Here's how the part is built. I have some questions about the finished solid (model axes, mm). Coordinates: 2 decimals unless noted, no trailing zeros. Loops run counter-clockwise (first coordinate to the right, second up) from the corner with the lowest first, then second, coordinate; pieces in that order, holes last. Notation, with made-up numbers: (24.5, -4) - (53.5, -4) arc R26 cw to (53.5, 25) - close; hole circle Ø5 at (16.25, 67). An arc over 180 degrees is marked (long way). Use a Markdown table: item, result.
```python
from build123d import *

# Parameters (mm, degrees)
SKETCH1_R           = 2
BOSS_EXTRUDE3_DEPTH = 5
FILLET9_R           = 10
FILLET10_R          = 3
FILLET11_R          = 3
FILLET12_R          = 3
FILLET13_R          = 0.5


with BuildPart() as part:
    # Sketch1 → Boss-Extrude3 (new body)
    with BuildSketch(Plane(origin=(0, 0, 0), x_dir=(1, 0, 0), z_dir=(0, 1, 0))):
        with BuildLine():
            Line((-4.046119318, 54.590604732), (-4.046119318, -7.195574606))
            ThreePointArc((-4.046119318, -7.195574606), (-11.635335702, -12.035866866), (-15.176119318, -20.311583503))
            ThreePointArc((-15.176119318, -20.311583503), (-15.239015435, -21.109389908), (-15.26, -21.909396551))
            ThreePointArc((-15.26, -21.909396551), (-15.239086668, -22.708042569), (-15.17640413, -23.504499555))
            Line((-15.17640413, -23.504499555), (-16.906872391, -23.686379161))
            ThreePointArc((-16.906872391, -23.686379161), (-18.44583537, -24.118938522), (-19.753766933, -25.038084689))
            ThreePointArc((-19.753766933, -25.038084689), (-19.56295199, -26.067629867), (-19.318516287, -27.085777598))
            ThreePointArc((-19.318516287, -27.085777598), (-17.749810888, -27.393475541), (-16.167960532, -27.162685373))
            Line((-16.167960532, -27.162685373), (-14.513122101, -26.624995641))
            ThreePointArc((-14.513122101, -26.624995641), (-14.246436916, -27.378091201), (-13.940703236, -28.116197446))
            ThreePointArc((-13.940703236, -28.116197446), (-13.596759365, -28.837290674), (-13.215547785, -29.539395055))
            Line((-13.215547785, -29.539395055), (-14.722432114, -30.409395176))
            ThreePointArc((-14.722432114, -30.409395176), (-15.952407023, -31.430510437), (-16.773411552, -32.802175926))
            ThreePointArc((-16.773411552, -32.802175926), (-16.180339688, -33.665100824), (-15.542918581, -34.49580411))
            ThreePointArc((-15.542918581, -34.49580411), (-13.984682857, -34.138850219), (-12.633461458, -33.284616422))
            Line((-12.633461458, -33.284616422), (-11.340389428, -32.120328997))
            ThreePointArc((-11.340389428, -32.120328997), (-10.790448835, -32.699845394), (-10.210932372, -33.249785918))
            ThreePointArc((-10.210932372, -33.249785918), (-9.603428978, -33.768642793), (-8.969603297, -34.25499435))
            Line((-8.969603297, -34.25499435), (-9.99234972, -35.66268407))
            ThreePointArc((-9.99234972, -35.66268407), (-10.700662735, -37.095795135), (-10.892781095, -38.682806536))
            ThreePointArc((-10.892781095, -38.682806536), (-9.999999818, -39.229903609), (-9.079809202, -39.729526311))
            ThreePointArc((-9.079809202, -39.729526311), (-7.80147625, -38.769641154), (-6.914522249, -37.439668504))
            Line((-6.914522249, -37.439668504), (-6.20680051, -35.850099247))
            ThreePointArc((-6.20680051, -35.850099247), (-5.468694229, -36.155832838), (-4.715598637, -36.422517933))
            ThreePointArc((-4.715598637, -36.422517933), (-3.94957857, -36.649423393), (-3.172733001, -36.835927528))
            Line((-3.172733001, -36.835927528), (-3.534499379, -38.53790452))
            ThreePointArc((-3.534499379, -38.53790452), (-3.598676752, -40.135213481), (-3.128689936, -41.66316212))
            ThreePointArc((-3.128689936, -41.66316212), (-2.09056923, -41.799833318), (-1.046718412, -41.881986139))
            ThreePointArc((-1.046718412, -41.881986139), (-0.269323601, -40.48514257), (6.05e-07, -38.909395406))
            Line((6.05e-07, -38.909395406), (5.43e-07, -37.169395268))
            ThreePointArc((5.43e-07, -37.169395268), (0.798647238, -37.14848194), (1.595104896, -37.085799334))
            ThreePointArc((1.595104896, -37.085799334), (2.387189815, -36.981519365), (3.172731623, -36.835927821))
            Line((3.172731623, -36.835927821), (3.534497981, -38.537904817))
            ThreePointArc((3.534497981, -38.537904817), (4.1255531, -40.023222459), (5.176380106, -41.22791215))
            ThreePointArc((5.176380106, -41.22791215), (6.180339749, -40.930525784), (7.167359489, -40.581003755))
            ThreePointArc((7.167359489, -40.581003755), (7.309397542, -38.988728703), (6.914523355, -37.439668011))
            Line((6.914523355, -37.439668011), (6.206801502, -35.850098805))
            ThreePointArc((6.206801502, -35.850098805), (6.927895349, -35.506154662), (7.630000317, -35.124942746))
            ThreePointArc((7.630000317, -35.124942746), (8.311191417, -34.707508302), (8.969602158, -34.254995178))
            ThreePointArc((8.969602158, -34.254995178), (10.210932755, -33.249785573), (11.340390155, -32.12032819))
            ThreePointArc((11.340390155, -32.12032819), (11.859247485, -31.512824296), (12.345599442, -30.87899807))
            ThreePointArc((12.345599442, -30.87899807), (12.7981126, -30.220587353), (13.215547081, -29.539396275))
            ThreePointArc((13.215547081, -29.539396275), (13.940703446, -28.116196975), (14.513122436, -26.624994609))
            ThreePointArc((14.513122436, -26.624994609), (14.740028108, -25.8589739), (14.926532387, -25.08212767))
            ThreePointArc((14.926532387, -25.08212767), (13.533608818, -14.858931995), (5.953880682, -7.858811478))
            Line((5.953880682, -7.858811478), (5.953880682, 54.590604732))
            ThreePointArc((5.953880682, 54.590604732), (-0.92910996, 71.20761409), (-17.546119318, 78.090604732))
            Line((-17.546119318, 78.090604732), (-17.546119318, 68.090604732))
            ThreePointArc((-17.546119318, 68.090604732), (-8.000177772, 64.136546278), (-4.046119318, 54.590604732))
        make_face()
        with Locations((0, -21.909395268)):
            Circle(SKETCH1_R, mode=Mode.SUBTRACT)
        with Locations((-12.546119318, 72.402117863)):
            Circle(SKETCH1_R, mode=Mode.SUBTRACT)
    extrude(amount=BOSS_EXTRUDE3_DEPTH)

    # Fillet9
    fillet9_edges = [part.edges().sort_by_distance(p)[0] for p in [
        (5.953880682, 2.5, 7.858811478),
    ]]
    fillet(fillet9_edges, radius=FILLET9_R)

    # Fillet10
    fillet10_edges = [part.edges().sort_by_distance(p)[0] for p in [
        (-4.046119318, 2.5, 7.195574606),
    ]]
    fillet(fillet10_edges, radius=FILLET10_R)

    # Fillet11
    fillet11_edges = [part.edges().sort_by_distance(p)[0] for p in [
        (-17.546119318, 2.5, -78.090604732),
    ]]
    fillet(fillet11_edges, radius=FILLET11_R)

    # Fillet12
    fillet12_edges = [part.edges().sort_by_distance(p)[0] for p in [
        (-17.546119318, 2.5, -68.090604732),
    ]]
    fillet(fillet12_edges, radius=FILLET12_R)

    # Fillet13
    fillet13_edges = [part.edges().sort_by_distance(p)[0] for p in [
        (7.167359489, 2.5, 40.581003755),
        (5.176380106, 2.5, 41.22791215),
        (-1.046718412, 2.5, 41.881986139),
        (-3.128689936, 2.5, 41.66316212),
        (-9.079809202, 2.5, 39.729526311),
        (-10.892781095, 2.5, 38.682806536),
        (-15.542918581, 2.5, 34.49580411),
        (-16.773411552, 2.5, 32.802175926),
        (-19.318516287, 2.5, 27.085777598),
        (-19.753766933, 2.5, 25.038084689),
    ]]
    fillet(fillet13_edges, radius=FILLET13_R)


solid = part.part
```
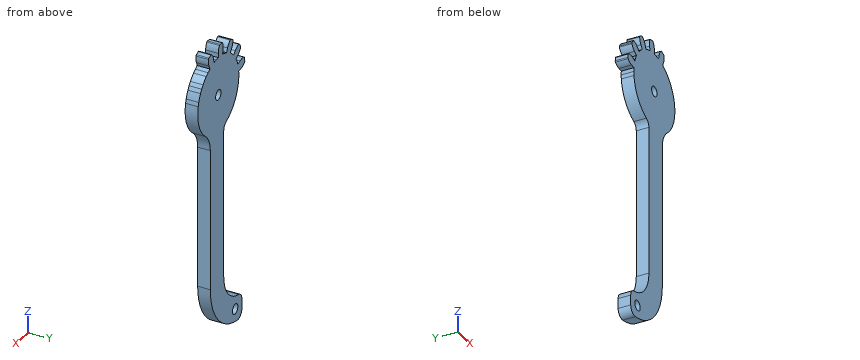
Q1. I want a section at B-B, the plane z = -42.5. Write out the boundary of the cut face in (x, y).
Check values:
| item | result |
|---|---|
| outline | (-4.05, 0) - (5.95, 0) - (5.95, 5) - (-4.05, 5) - close |
Q2. I want a section at C-C, the plane z = -64. Write out the boundary of the cut face in (x, y).
Check values:
| item | result |
|---|---|
| outline | (-7.87, 0) - (3.99, 0) - (3.99, 5) - (-7.87, 5) - close |
Q3. Will these pins go through, and if not, where does the flat tip stop? P1, Ø3, axis at x = 0.5, y = 0.5, coming from the -Z side; P2, Ø0.5, axis at y = 1.5, z = 38.5, coming from the +X side; P3, Ø1.2, axis at y = 3.5, z = -72.5, coming from the -X side.
Check values:
| item | result |
|---|---|
| P1 | z = -71.28 |
| P2 | x = 7.28 |
| P3 | x = -17.55 |
Q4. Please list where these lines run through material, in increasing order: L1, parallel to X at y = 1.25, z = -8.5; L2, parallel to X at y = 2.75, z = 37.5; L3, parallel to Z at x = -7, y = 4.25. Write a range as from..to.
Check values:
| item | result |
|---|---|
| L1 | -4.05..5.95 |
| L2 | -10.8..-6.94, -3.31..0, 3.31..6.94 |
| L3 | -75.59..-63.02, 8.35..37.62 |
Q5. I want a section at A-A, the plane y = 1.8. Give the number of separate pieces and of enclosed holes in the cut face, then the cut area to 3 significant figures.
Check values:
| item | result |
|---|---|
| separate pieces | 1 |
| enclosed holes | 2 |
| area | 1,690 mm^2 |
